Check sheet for the modelled part. Datum: model origin and axes. Units: mm. Face numbers are marked on the shaded views. A direction names the side the tool comes from. Coordinates: 2 decimals unless noted, no trailing zeros. Write each loop counter-clockwise with the first axis right and the second up, starting at its lowest first coordinate (ties: lowest second). Pieces come first, ordered by that corner, then holes. Notation, with made-up numbers: M 41,5 L 46,5 A29 ccw 46,41 Z; hole C -3.5,52 d10. An arc over 180 degrees is marked long. Answer as CSV lines item,"result". Start each with the question number.
Q1. Sectioned sample at B-B, the plane y = 4.63. Record the cut outline in (x, z), then the cut area to 3 significant figures.
Q2. Sectioned sample at D-D, the plane z = 28.2. Record the cut outline in (x, y) (3 decimals), then the cut area to 3 significant figures.
Q3. Thickness scan on line 1 along Y through (x, z) = (1.05, 51.77); line 2 along Y through (x, z) = (4, 4); line 3 along Z through (x, y) = (2, 51). Record the ranges inside material, lowest first. Write a range as from..to.
Q4. Sectioned sample at A-A, the plane z = 4.63. Record the cut outline in (x, y).
Q5. Depth check by flat-ended pin: pin 1 Ø2.5 at (y, z) = (53, 3) entering from +X; pin 2 Ø7 at (x, y) = (81, 50.5) entering from -Z; pin 3 Ø2.5 at (x, y) = (50, 5.5) entering from +Z; pin 4 Ø2.5 at (x, z) = (33, 51) entering from +Y. Enter the tip coordinate at first touch or a pass-through.
Q6. Access from +Z, -Z, +X, -X, +Y, -Y to the whole of each face (thin tool, end or side, straight path). Record for the marked faces 1, 2 and 3.
Q7. Sectioned sample at C-C, the plane x = 99. Record the cut outline in (y, z).
Q8. Mould release check, pull along Y, two halves, no side actions. Record for the marked faces 4, 5, 6 and 7: pulls with the +Y half, pulls with the -Y half, needs draft (parallel to the pull), parting line crosses it, or undercut.
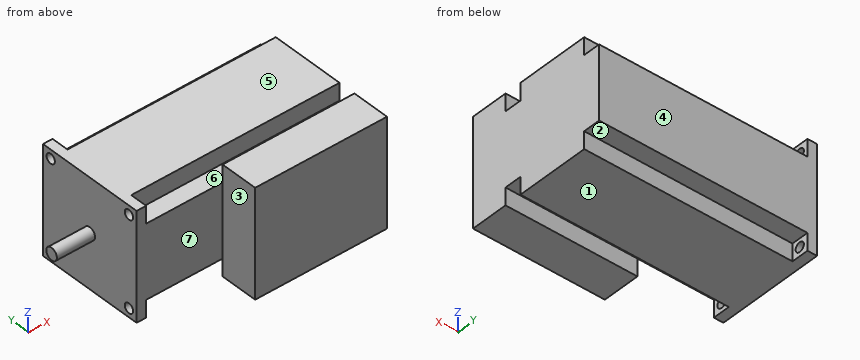
from build123d import *

# Parameters (mm, degrees)
BOSS_EXTRUDE1_DEPTH = 56.4
SKETCH2_R           = 2.5
CUT_EXTRUDE1_DEPTH  = 5
SKETCH3_R           = 3.175
BOSS_EXTRUDE2_DEPTH = 20
SKETCH4_W           = 9
SKETCH4_H           = 9
CUT_EXTRUDE2_DEPTH  = 109


with BuildPart() as part:
    # Sketch1 → Boss-Extrude1 (new body)
    with BuildSketch(Plane.XY):
        Polygon((45, 0), (45, -19.6), (114, -19.6), (114, 0), (114, 56.4), (0, 56.4), (0, 0), align=None)
    extrude(amount=BOSS_EXTRUDE1_DEPTH)

    # Sketch2 → Cut-Extrude1 (cut)
    with BuildSketch(Plane.ZY):
        with Locations((4.63, 4.63)):
            Circle(SKETCH2_R)
        with Locations((51.77, 4.63)):
            Circle(SKETCH2_R)
        with Locations((51.77, 51.77)):
            Circle(SKETCH2_R)
        with Locations((4.63, 51.77)):
            Circle(SKETCH2_R)
    extrude(amount=-CUT_EXTRUDE1_DEPTH, mode=Mode.SUBTRACT)

    # Sketch3 → Boss-Extrude2 (add)
    with BuildSketch(Plane.ZY):
        with Locations(Location((28.2, 28.2, 0), (0, 0, 180))):
            Circle(SKETCH3_R)
    extrude(amount=BOSS_EXTRUDE2_DEPTH)

    # Sketch4 → Cut-Extrude2 (cut)
    with BuildSketch(Plane(origin=(114, 0, 0), x_dir=(0, 0, -1), z_dir=(1, 0, 0))):
        with Locations((-51.9, 51.9)):
            Rectangle(SKETCH4_W, SKETCH4_H)
        with Locations((-4.5, 51.9)):
            Rectangle(SKETCH4_W, SKETCH4_H)
        with Locations((-4.5, 4.5)):
            Rectangle(SKETCH4_W, SKETCH4_H)
        with Locations((-51.9, 4.5)):
            Rectangle(SKETCH4_W, SKETCH4_H)
    extrude(amount=-CUT_EXTRUDE2_DEPTH, mode=Mode.SUBTRACT)


solid = part.part
Output:
1,outline,"M 0,0 L 5,0 L 5,2.13 L 0,2.13 Z; M 0,7.13 L 5,7.13 L 5,9 L 114,9 L 114,47.4 L 5,47.4 L 5,49.27 L 0,49.27 Z; M 0,54.27 L 5,54.27 L 5,56.4 L 0,56.4 Z"
1,area,"4,420 mm^2"
2,outline,"M -20,25.025 L 0,25.025 L 0,0 L 45,0 L 45,-19.6 L 114,-19.6 L 114,56.4 L 0,56.4 L 0,31.375 L -20,31.375 Z"
2,area,"7,910 mm^2"
3,line 1,"y = 0..2.13, 7.13..49.27, 54.27..56.4"
3,line 2,"y = 0..2.21, 7.05..49.35, 54.19..56.4"
3,line 3,"z = 0..2.25, 7.01..49.39, 54.15..56.4"
4,outline,"M 0,0 L 5,0 L 5,2.13 L 0,2.13 Z; M 0,7.13 L 5,7.13 L 5,9 L 114,9 L 114,47.4 L 5,47.4 L 5,49.27 L 0,49.27 Z; M 0,54.27 L 5,54.27 L 5,56.4 L 0,56.4 Z; M 45,-19.6 L 114,-19.6 L 114,0 L 45,0 Z"
5,pin 1,"stops at x = 5"
5,pin 2,"stops at z = 0"
5,pin 3,"stops at z = 47.4"
5,pin 4,"stops at y = 47.4"
6,face 1,"-Z, +X, -X, +Y, -Y"
6,face 2,"-Z, +X, +Y"
6,face 3,"+Z, -Z, -X, -Y"
7,outline,"M -19.6,0 L 0,0 L 0,9 L 9,9 L 9,0 L 47.4,0 L 47.4,9 L 56.4,9 L 56.4,47.4 L 47.4,47.4 L 47.4,56.4 L 9,56.4 L 9,47.4 L 0,47.4 L 0,56.4 L -19.6,56.4 Z"
8,face 4,"pulls with the +Y half"
8,face 5,"needs draft"
8,face 6,"undercut"
8,face 7,"pulls with the -Y half"
